from build123d import *

# Parameters (mm, degrees)
PAD007_DEPTH         = 10
SKETCH017_W          = 29
SKETCH017_H          = 10
PAD008_DEPTH         = 30
SKETCH018_R          = 1.6
POCKET007_DEPTH      = 0.001
POCKET007_DEPTH_BACK = 94.001
PAD009_DEPTH         = 29
SKETCH020_R          = 2.5
PAD010_DEPTH         = 10
POCKET008_DEPTH      = 10.001


with BuildPart() as part:
    # Sketch016 → Pad007 (new body)
    with BuildSketch(Plane.XZ):
        with BuildLine():
            ThreePointArc((9.5, 90), (4.995983, 93.968119), (1.627017, 89))
            Line((-1.627017, 89), (1.627017, 89))
            ThreePointArc((-1.627017, 89), (-4.995983, 93.968119), (-9.5, 90))
            Line((-9.5, 90), (-14.5, 90))
            Line((-14.5, 90), (-14.5, 0))
            Line((-14.5, 0), (14.5, 0))
            Line((14.5, 90), (14.5, 0))
            Line((9.5, 90), (14.5, 90))
        make_face()
        Polygon((9.5, 90), (14.5, 90), align=None)
    extrude(amount=PAD007_DEPTH)

    # Sketch017 (on Face10 of Pad007) → Pad008 (join)
    with BuildSketch(Plane.XZ.offset(10)):
        with Locations((0, 5)):
            Rectangle(SKETCH017_W, SKETCH017_H)
    extrude(amount=PAD008_DEPTH)

    # Sketch018 → Pocket007 (cut, two sides)
    with BuildSketch(Plane.XY) as pocket007_sk:
        with Locations((-4, -25)):
            Circle(SKETCH018_R)
        with Locations((4, -35)):
            Circle(SKETCH018_R)
    extrude(amount=-POCKET007_DEPTH, mode=Mode.SUBTRACT)
    extrude(pocket007_sk.sketch, amount=POCKET007_DEPTH_BACK, mode=Mode.SUBTRACT)

    # Sketch019 (on Face3 of Pocket007) → Pad009 (join)
    with BuildSketch(Plane(origin=(14.5, 0, 0), x_dir=(0, 0, 1), z_dir=(1, 0, 0))):
        Polygon((10, 17.517339), (17.517341, 10), (10, 10), align=None)
    extrude(amount=-PAD009_DEPTH)

    # Sketch020 (on Face4 of Pad009) → Pad010 (join)
    with BuildSketch(Plane.XZ.offset(10)):
        with Locations((-5.5, 90)):
            Circle(SKETCH020_R)
        with Locations((5.5, 90)):
            Circle(SKETCH020_R)
    extrude(amount=PAD010_DEPTH)

    # Sketch021 (on Face5 of Pad010) → Pocket008 (cut, through all)
    with BuildSketch(Plane.XZ.offset(10)):
        with BuildLine():
            ThreePointArc((8, 70), (0, 78), (-8, 70))
            Line((-8, 70), (-8, 37.517341))
            ThreePointArc((-8, 37.517341), (0, 29.517341), (8, 37.517341))
            Line((8, 70), (8, 37.517341))
        make_face()
    extrude(amount=-POCKET008_DEPTH, mode=Mode.SUBTRACT)


solid = part.part
Can you work these out from the model? Positions are in its coordinate system, mm. A direction names the side the tool comes from. Give positions to 0.01 mm unless a question says otherwise; leave off trailing zeros. Loops run counter-clockwise (first coordinate to the right, second up) from the corner with the lowest first, then second, coordinate; pieces in that order, holes last. Notation, with made-up numbers: M 84.5,-35 L 133.5,-35 A15 ccw 133.5,-18 Z; hole C 32,-19 d11. An arc over 180 degrees is marked long. One line per item, written item: value.
1) Imagine slicing it at C-C on x = 4. Write out the boundary of the cut face in (y, z), and give its area (3 significant figures).
Geometry check:
outline: M -40,0 L -36.6,0 L -36.6,10 L -40,10 Z; M -33.4,0 L 0,0 L 0,30.59 L -10,30.59 L -10,17.52 L -17.52,10 L -33.4,10 Z; M -20,88 L -10,88 L -10,76.93 L 0,76.93 L 0,93.71 L -10,93.71 L -10,92 L -20,92 Z
area: 810 mm²
2) On a 3-axis mill with a long thin cutter (end or side, diameter ignored), from which of +Z, -Z, +X, -X, +Y, -Y can I reach the whole of each face in a straight line? I mean faces 1 (the face through (-5.83, -14.93, 92.48)), 2 (the face through (0, -5, 78)), 3 (the face through (5, -20, 90)), 4 (the face through (0.2, -13.81, 13.71)), 5 (the face through (12, -5, 90)). Say none if no direction works.
Geometry check:
face 1: -Y
face 2: +Y, -Y
face 3: +Z, +X, -X, -Y
face 4: +X, -X, -Y
face 5: +Z, +X, +Y, -Y
3) Thinking about a two-plate mould opening in X: for faces 6 (the face through (-4.902, -4.93, 93.955)), 7 (the face through (14.5, -9.7, 35.2)), 8 (the face through (0, -20, 0)), which applies, +X half, -X half, draft (parallel to the pull), parting line (faces both ways), or undercut?
Geometry check:
face 6: undercut
face 7: +X half
face 8: draft
4) Imagine slicing it at B-B on z = 34. Write out the boundary of the cut face in (x, y).
Geometry check:
outline: M -14.5,-10 L -7.19,-10 L -7.19,0 L -14.5,0 Z; M 7.19,-10 L 14.5,-10 L 14.5,0 L 7.19,0 Z
5) Imagine slicing it at D-D on x = -11.75. Write out the boundary of the cut face in (y, z), and give its area (3 significant figures).
Geometry check:
outline: M -40,0 L 0,0 L 0,90 L -10,90 L -10,17.52 L -17.52,10 L -40,10 Z
area: 1,230 mm²
6) Imagine slicing it at A-A on y = -25. Write out the boundary of the cut face in (x, z), and give its area (3 significant figures).
Geometry check:
outline: M -14.5,0 L -5.6,0 L -5.6,10 L -14.5,10 Z; M -2.4,0 L 14.5,0 L 14.5,10 L -2.4,10 Z
area: 258 mm²
7) Please list where these lines run through material, in increasing order: line 1 (X direction, y = -35, z = 4.75); line 2 (Y direction, x = -4, z = 3.5); line 3 (X direction, y = -25, z = 3).
Geometry check:
line 1: x = -14.5 to 2.4, 5.6 to 14.5
line 2: y = -40 to -26.6, -23.4 to 0
line 3: x = -14.5 to -5.6, -2.4 to 14.5
8) I'm going to push flat-ended pins straight in: pin 1 (8 mm diameter, centred on x = -0.5, z = 19, fed in from -Y); pin 2 (1.5 mm diameter, centred on x = 3.5, y = -28, fed in from -Z); pin 3 (4 mm diameter, centred on x = 6, z = 90, fed in from -Y); pin 4 (8 mm diameter, centred on x = -9, z = 63.5, fed in from -Y). Where does each tip first touch, or does it pass through?
Geometry check:
pin 1: stops at y = -12.52
pin 2: stops at z = 0
pin 3: stops at y = -20
pin 4: stops at y = -10
